The listing builds one solid part. Answer for the finished solid, in the listing's coordinates (mm). Coordinates: 2 decimals unless noted, no trailing zeros. Loops run counter-clockwise (first coordinate to the right, second up) from the corner with the lowest first, then second, coordinate; pieces in that order, holes last. Notation, with made-up numbers: M 7.5,-30 L 19.5,-30 A19 cw 19.5,3 Z; hole C -14.5,-25 d8. An arc over 180 degrees is marked long. Answer in a Markdown table with one row per item. Add a question column.
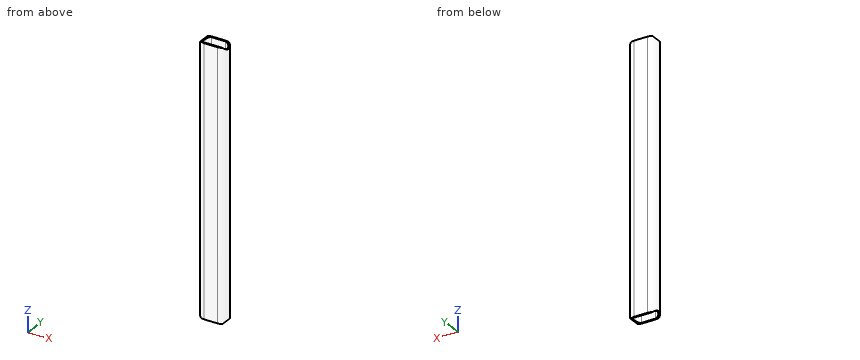
from build123d import *

# Parameters (mm, degrees)
EXTRUDE_1_DEPTH          = 292
CUT_EXTRUDE_1_DEPTH      = 293.961601579
CUT_EXTRUDE_1_DEPTH_BACK = 293.961601579
SKETCH_2_R               = 7.5


with BuildPart() as part:
    # Эскиз1 → Бобышка-Вытянуть1 (new body)
    with BuildSketch(Plane.XY):
        with BuildLine():
            Line((0, 7.5), (15, 7.5))
            ThreePointArc((15, 7.5), (22.5, 0), (15, -7.5))
            Line((15, -7.5), (0, -7.5))
            ThreePointArc((0, -7.5), (-7.5, 0), (0, 7.5))
        make_face()
        with BuildLine():
            Line((0, 6), (15, 6))
            ThreePointArc((15, 6), (21, 0), (15, -6))
            Line((15, -6), (0, -6))
            ThreePointArc((0, -6), (-6, 0), (0, 6))
        make_face(mode=Mode.SUBTRACT)
    extrude(amount=EXTRUDE_1_DEPTH)

    # Эскиз2 → Вырез-Вытянуть1 (cut, two sides: drawn at the far end of the back side and taken through both)
    with BuildSketch(Plane(origin=(0, 0, 0), x_dir=(0, 0, -1), z_dir=(1, 0, 0)).offset(-CUT_EXTRUDE_1_DEPTH_BACK)):
        with Locations((4.5, 0)):
            Circle(SKETCH_2_R)
        with Locations((-296.5, 0)):
            Circle(SKETCH_2_R)
    extrude(amount=CUT_EXTRUDE_1_DEPTH + CUT_EXTRUDE_1_DEPTH_BACK, mode=Mode.SUBTRACT)


solid = part.part
(1) A cutting plane is placed at A-A (y = 0). Give the vertices of the cut face in (x, z).
(2) A cutting plane is placed at C-C (x = 7.5). Give the vertices of the cut face in (y, z), plus the area to 3 significant figures.
(3) Each of these flat-tipped pins is pushed along its axis until it touches: pin 1 (1 mm diameter, centred on y = -2, z = 262.5, fed in from +X); pin 2 (3 mm diameter, centred on y = -4.5, z = 91, fed in from +X); pin 3 (5 mm diameter, centred on y = 5, z = 57, fed in from +X); pin 4 (1.5 mm diameter, centred on x = 5.5, y = 3.5, fed in from +Z). Where does it stop, or does it pass through?
(4) Straight lines are drawn through the part: line 1 (Y direction, x = 5, z = 34); line 2 (X direction, y = 0.75, z = 217); line 3 (X direction, y = -5.25, z = 20). For each, find the intervals that lie inside material, in ascending order.
(5) A cutting plane is placed at B-B (z = 30). Give the vertices of the cut face in (x, y).
Solved:
| question | item | result |
|---|---|---|
| 1 | outline | M -7.5,3 L -6,3 L -6,289 L -7.5,289 Z; M 21,3 L 22.5,3 L 22.5,289 L 21,289 Z |
| 2 | outline | M -7.5,0 L -6,0 L -6,292 L -7.5,292 Z; M 6,0 L 7.5,0 L 7.5,292 L 6,292 Z |
| 2 | area | 876 mm² |
| 3 | pin 1 | stops at x = 22.35 |
| 3 | pin 2 | stops at x = 21.87 |
| 3 | pin 3 | stops at x = 22.07 |
| 3 | pin 4 | passes through |
| 4 | line 1 | y = -7.5 to -6, 6 to 7.5 |
| 4 | line 2 | x = -7.46 to -5.95, 20.95 to 22.46 |
| 4 | line 3 | x = -5.36 to -2.9, 17.9 to 20.36 |
| 5 | outline | M 0,-7.5 L 15,-7.5 A7.5 ccw 15,7.5 L 0,7.5 A7.5 ccw Z; hole M 0,-6 L 15,-6 A6 ccw 15,6 L 0,6 A6 ccw Z |
